The listing builds one solid part. Answer for the finished solid, in the listing's coordinates (mm). Face numbers are marked on the shaded views. A direction names the side the tool comes from. Give positions to 0.01 mm unless a question says otherwise; leave off trailing zeros. Write each loop counter-clockwise with the first axis right and the second up, starting at its lowest first coordinate (ties: lowest second). Pieces come first, ordered by that corner, then holes. Notation, with made-up numbers: (-6.75, -26) - (40.25, -26) arc R18 cw to (40.25, 0) - close; hole circle Ø4 at (-28, 36). An arc over 180 degrees is marked (long way). One line per question, with ' | ' between items. Start each with the question number.
1. A cutting plane is placed at C-C (x = 15). Determine the outline of the cut face in (y, z).
2. A cutting plane is placed at B-B (z = 16). Determine the outline of the cut face in (x, y).
3. The mould has two halves that part along Y. Classify the marked faces 4, 5 and 6: +Y half, -Y half, draft (parallel to the pull), parting line (faces both ways), or undercut.
4. Given P1, Ø2, axis at x = 26.5, z = 34.5, coming from the -Y side; P2, Ø1, axis at y = -6, z = 33.5, coming from the -X side; P3, Ø6, axis at x = 15, z = 16, coming from the -Y side; P4, Ø12, axis at y = -35.5, z = 29.5, coming from the -X side, each flat-ended and moving along its own axis, determine where each tip first touches the part or whether it passes through.
5. Find the intervals of material crossed by L1, parallel to Y at x = 19, z = 33.5; L2, parallel to X at y = 1, z = 16; L3, parallel to X at y = -13.5, z = 17.5, in increasing order. Write a range as from..to.
6. A cutting plane is placed at D-D (y = 1.5). Determine the outline of the cut face in (x, z), then the cut area to 3 significant figures.
7. A cutting plane is placed at A-A (y = -30). Determine the outline of the cut face in (x, z).
8. For the marked faces 1, 2 and 3, determine the directions among +Z, -Z, +X, -X, +Y, -Y from which every point of the face is accessible in a straight line to the end or side of a thin tool.
```python
from build123d import *

# Parameters (mm, degrees)
BOSS_EXTRUDE1_DEPTH = 60
FILLET1_R           = 5
SKETCH2_R           = 5
CUT_EXTRUDE1_DEPTH  = 75
SKETCH3_W           = 2.5
SKETCH3_H           = 60
BOSS_EXTRUDE2_DEPTH = 15


with BuildPart() as part:
    # Sketch1 → Boss-Extrude1 (new body)
    with BuildSketch(Plane.XY):
        Polygon((0, 0), (35, 0), (35, -20), (0, -20), (0, -25), (40, -25), (40, 5), (0, 5), align=None)
    extrude(amount=BOSS_EXTRUDE1_DEPTH)

    # Fillet1
    fillet1_edges = [part.edges().sort_by_distance(p)[0] for p in [
        (35, -20, 30),
        (35, 0, 30),
    ]]
    fillet(fillet1_edges, radius=FILLET1_R)

    # Sketch2 → Cut-Extrude1 (cut)
    with BuildSketch(Plane(origin=(0, 5, 0), x_dir=(1, 0, 0), z_dir=(0, 1, 0))):
        with Locations(Location((15, -44, 0), (0, 0, 180))):
            Circle(SKETCH2_R)
        with Locations(Location((15, -16, 0), (0, 0, 270))):
            Circle(SKETCH2_R)
    extrude(amount=-CUT_EXTRUDE1_DEPTH, mode=Mode.SUBTRACT)

    # Sketch3 → Boss-Extrude2 (add)
    with BuildSketch(Plane.XZ.offset(25)):
        with Locations((31.25, 30)):
            Rectangle(SKETCH3_W, SKETCH3_H)
        with Locations((38.75, 30)):
            Rectangle(SKETCH3_W, SKETCH3_H)
    extrude(amount=BOSS_EXTRUDE2_DEPTH)


solid = part.part
```
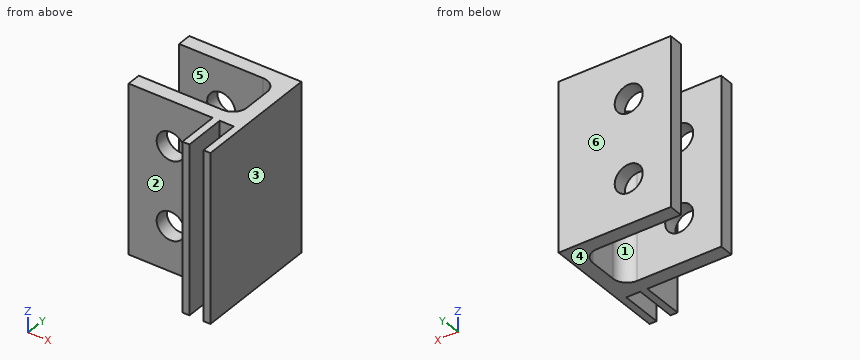
Determined:
1) outline: (-25, 0) - (-20, 0) - (-20, 11) - (-25, 11) - close; (-25, 21) - (-20, 21) - (-20, 39) - (-25, 39) - close; (-25, 49) - (-20, 49) - (-20, 60) - (-25, 60) - close; (0, 0) - (5, 0) - (5, 11) - (0, 11) - close; (0, 21) - (5, 21) - (5, 39) - (0, 39) - close; (0, 49) - (5, 49) - (5, 60) - (0, 60) - close
2) outline: (0, -25) - (10, -25) - (10, -20) - (0, -20) - close; (0, 0) - (10, 0) - (10, 5) - (0, 5) - close; (20, -25) - (30, -25) - (30, -40) - (32.5, -40) - (32.5, -25) - (37.5, -25) - (37.5, -40) - (40, -40) - (40, 5) - (20, 5) - (20, 0) - (30, 0) arc R5 cw to (35, -5) - (35, -15) arc R5 cw to (30, -20) - (20, -20) - close
3) face 4: draft | face 5: undercut | face 6: +Y half
4) P1: y = -25 | P2: x = 35 | P3: through | P4: x = 30
5) L1: -25..-20, 0..5 | L2: 0..10, 20..40 | L3: 35..40
6) outline: (0, 0) - (40, 0) - (40, 60) - (0, 60) - close; hole circle Ø10 at (15, 16); hole circle Ø10 at (15, 44) | area: 2,240 mm2
7) outline: (30, 0) - (32.5, 0) - (32.5, 60) - (30, 60) - close; (37.5, 0) - (40, 0) - (40, 60) - (37.5, 60) - close
8) face 1: +Z, -Z, -X | face 2: +Z, -Z, -X, -Y | face 3: +Z, -Z, +X, +Y, -Y
